Can you work these out from the model? Positions are in its coordinate system, mm. A direction names the side the tool comes from. Coordinates: 2 decimals unless noted, no trailing zeros. Order: outer loops, then holes, each group sorted by start corner. A loop starts at its lowest first (then second) coordinate and runs counter-clockwise, first axis right, second up. Notation, with made-up numbers: (-21, 59) -> (14, 59) arc R19 ccw to (14, 69) -> close; hole circle Ø10 at (39, 30). An arc over 180 degrees is marked (long way). Answer in a Markdown table with one row per item. Add a question column.
1. If I drill on line 1 along Z through (x, y) = (-0.5, -6.5) (3 decimals); line 2 along Z through (x, y) = (-2, -5.5) (3 decimals); line 3 along Y through (x, z) = (-1, 123.5), over which ranges is the centre line in solid material (lowest first)? Write a range as [from, to].
2. Will these pins go through, and if not, where does the flat tip stop? pin 1 (1.5 mm diameter, centred on x = 3.5, z = 153, fed in from +Y); pin 2 (5 mm diameter, centred on x = -6.5, z = 179, fed in from -Y); pin 3 (0.6 mm diameter, centred on y = -8.5, z = 171.5, fed in from -X); pin 4 (4 mm diameter, centred on x = 0, z = 140.716, fed in from -Y).
3. Imagine slicing it at A-A on y = 0. Write out the boundary of the cut face in (x, z) (3 decimals).
4. On a 3-axis mill with a long thin cutter (end or side, diameter ignored), from which of +Z, -Z, +X, -X, +Y, -Y can I reach the whole of each face in a straight line? I mean faces 1 (the face through (4, 0, 570.865)), 2 (the face through (0, 0, 0)). Say none if no direction works.
5. Imagine slicing it at C-C on x = 6.5. Write out the boundary of the cut face in (y, z) (3 decimals), plus the area to 3 significant figures.
6. Imagine slicing it at B-B on z = 217. Write out the boundary of the cut face in (x, y) (3 decimals), plus the area to 3 significant figures.
from build123d import *

# Parameters (mm, degrees)
SKETCH1_R           = 9.525
BOSS_EXTRUDE1_DEPTH = 586.105
CUT_EXTRUDE2_REACH  = 588.492
SKETCH3_R           = 3.175
CUT_EXTRUDE3_DEPTH  = 2.38125
SKETCH6_OUTSIDE_W   = 138.394
SKETCH6_OUTSIDE_H   = 138.394
SKETCH6_OUTSIDE_R   = 3.175
CUT_EXTRUDE4_DEPTH  = 15.24


with BuildPart() as part:
    # Sketch1 → Boss-Extrude1 (new body)
    with BuildSketch(Plane.XY):
        Circle(SKETCH1_R)
    extrude(amount=BOSS_EXTRUDE1_DEPTH)

    # Sketch3 → Cut-Extrude2 (cut, up to next)
    with BuildSketch(Plane(origin=(0, -9.525, 0), x_dir=(1, 0, 0), z_dir=(0, 1, 0)), mode=Mode.PRIVATE) as cut_extrude2_sk1:
        with Locations(Location((0, -445.389, 0), (0, 0, 90))):
            Circle(SKETCH3_R)
    cut_extrude2_tool1 = extrude(cut_extrude2_sk1.sketch, amount=CUT_EXTRUDE2_REACH, mode=Mode.PRIVATE) & part.part
    # Sketch3 → Cut-Extrude2 (cut, up to next)
    with BuildSketch(Plane(origin=(0, -9.525, 0), x_dir=(1, 0, 0), z_dir=(0, 1, 0)), mode=Mode.PRIVATE) as cut_extrude2_sk2:
        with Locations(Location((0, -140.716, 0), (0, 0, 90))):
            Circle(SKETCH3_R)
    cut_extrude2_tool2 = extrude(cut_extrude2_sk2.sketch, amount=CUT_EXTRUDE2_REACH, mode=Mode.PRIVATE) & part.part
    add(cut_extrude2_tool1.solids().sort_by_distance((0, -9.525, 445.389))[0], mode=Mode.SUBTRACT)
    add(cut_extrude2_tool2.solids().sort_by_distance((0, -9.525, 140.716))[0], mode=Mode.SUBTRACT)

    # Sketch5 → Cut-Extrude3 (cut)
    with BuildSketch(Plane(origin=(0, -9.525, 0), x_dir=(1, 0, 0), z_dir=(0, 1, 0))):
        with BuildLine():
            Line((-2.38125, -178.816), (-2.38125, -159.766))
            ThreePointArc((-2.38125, -159.766), (0, -157.38475), (2.38125, -159.766))
            Line((2.38125, -159.766), (2.38125, -178.816))
            ThreePointArc((2.38125, -178.816), (0, -181.19725), (-2.38125, -178.816))
        make_face()
        with BuildLine():
            Line((2.38125, -407.289), (2.38125, -426.339))
            ThreePointArc((2.38125, -426.339), (0, -428.72025), (-2.38125, -426.339))
            Line((-2.38125, -426.339), (-2.38125, -407.289))
            ThreePointArc((-2.38125, -407.289), (0, -404.90775), (2.38125, -407.289))
        make_face()
    extrude(amount=CUT_EXTRUDE3_DEPTH, mode=Mode.SUBTRACT)

    # Sketch6 outside → Cut-Extrude4 (cut)
    with BuildSketch(Plane.XY.offset(586.105)):
        Rectangle(SKETCH6_OUTSIDE_W, SKETCH6_OUTSIDE_H)
        Circle(SKETCH6_OUTSIDE_R, mode=Mode.SUBTRACT)
    extrude(amount=-CUT_EXTRUDE4_DEPTH, mode=Mode.SUBTRACT)


solid = part.part
Answers follow:
| question | item | result |
|---|---|---|
| 1 | line 1 | z = [0, 137.581], [143.851, 442.254], [448.524, 570.865] |
| 1 | line 2 | z = [0, 138.25], [143.182, 442.923], [447.855, 570.865] |
| 1 | line 3 | y = [-9.47, 9.47] |
| 2 | pin 1 | stops at y = 9.12 |
| 2 | pin 2 | stops at y = -8.64 |
| 2 | pin 3 | stops at x = -4.85 |
| 2 | pin 4 | passes through |
| 3 | outline | (-9.525, 0) -> (9.525, 0) -> (9.525, 570.865) -> (3.175, 570.865) -> (3.175, 586.105) -> (-3.175, 586.105) -> (-3.175, 570.865) -> (-9.525, 570.865) -> close; hole circle Ø6.35 at (0, 140.716); hole circle Ø6.35 at (0, 445.389) |
| 4 | face 1 | +Z |
| 4 | face 2 | -Z, +X, -X, +Y, -Y |
| 5 | outline | (-6.962, 0) -> (6.962, 0) -> (6.962, 570.865) -> (-6.962, 570.865) -> close |
| 5 | area | 7,950 mm² |
| 6 | outline | circle Ø19.05 at (0, 0) |
| 6 | area | 285 mm² |
